Check sheet for the modelled part. Datum: model origin and axes. Units: mm. A direction names the side the tool comes from. Round coordinates to 2 decimals unless told otherwise and drop trailing zeros. Write each loop counter-clockwise with the first axis right and the second up, starting at its lowest first coordinate (ties: lowest second). Pieces come first, ordered by that corner, then holes. Notation, with made-up numbers: (80, 77) -> (106, 77) arc R25 cw to (106, 109) -> close; hole circle Ø1 at (-1.75, 23.25). An arc over 180 degrees is marked (long way). One line per item, written item: value.
from build123d import *

# Parameters (mm, degrees)
SKETCH1_W           = 99.695
SKETCH1_H           = 17.526
BOSS_EXTRUDE1_DEPTH = 2.54
SKETCH2_W           = 104.14
SKETCH2_H           = 20.193
BOSS_EXTRUDE2_DEPTH = 2.54
SKETCH4_W           = 20.32
SKETCH4_H           = 8.89
BOSS_EXTRUDE3_DEPTH = 3.81
SKETCH5_W           = 50.8
SKETCH5_H           = 17.526
CUT_EXTRUDE1_DEPTH  = 54.282554483


with BuildPart() as part:
    # Sketch1 → Boss-Extrude1 (new body)
    with BuildSketch(Plane(origin=(0, 0, 0), x_dir=(1, 0, 0), z_dir=(0, 1, 0))):
        Rectangle(SKETCH1_W, SKETCH1_H)
    extrude(amount=BOSS_EXTRUDE1_DEPTH)

    # Sketch2 → Boss-Extrude2 (add)
    with BuildSketch(Plane(origin=(0, 2.54, 0), x_dir=(1, 0, 0), z_dir=(0, 1, 0))):
        Rectangle(SKETCH2_W, SKETCH2_H)
    extrude(amount=BOSS_EXTRUDE2_DEPTH)

    # Sketch4 → Boss-Extrude3 (add)
    with BuildSketch(Plane(origin=(0, 5.08, 0), x_dir=(1, 0, 0), z_dir=(0, 1, 0))):
        with Locations((28.80358553, 0)):
            Rectangle(SKETCH4_W, SKETCH4_H)
    extrude(amount=BOSS_EXTRUDE3_DEPTH)

    # Sketch5 → Cut-Extrude1 (cut, through all)
    with BuildSketch(Plane(origin=(0, 5.08, 0), x_dir=(1, 0, 0), z_dir=(0, 1, 0))):
        with Locations((-21.59, 0)):
            Rectangle(SKETCH5_W, SKETCH5_H)
    extrude(amount=-CUT_EXTRUDE1_DEPTH, mode=Mode.SUBTRACT)


solid = part.part
Item 1: Sectioned sample at B-B on x = -41.5. Enter the section's corners in (y, z).
Answer:
outline: (2.54, -10.1) -> (5.08, -10.1) -> (5.08, -8.76) -> (2.54, -8.76) -> close; (2.54, 8.76) -> (5.08, 8.76) -> (5.08, 10.1) -> (2.54, 10.1) -> close
Item 2: Mould release check, pull along Z, two halves, no side actions. Record for faces 1 (the flat face through (29, 7, -4.445)), 2 (the flat face through (-22, 4, 8.763)), 3 (the flat face through (18.644, 7, 0)): pulls with the +Z half, pulls with the -Z half, needs draft (parallel to the pull), parting line crosses it, or undercut.
Answer:
face 1: pulls with the -Z half
face 2: undercut
face 3: needs draft
Item 3: Sectioned sample at A-A on z = -1.25. Enter the section's corners in (x, y), and give its area (3 significant figures).
Answer:
outline: (-52.07, 2.54) -> (-49.85, 2.54) -> (-49.85, 0) -> (-46.99, 0) -> (-46.99, 5.08) -> (-52.07, 5.08) -> close; (3.81, 0) -> (49.85, 0) -> (49.85, 2.54) -> (52.07, 2.54) -> (52.07, 5.08) -> (38.96, 5.08) -> (38.96, 8.89) -> (18.64, 8.89) -> (18.64, 5.08) -> (3.81, 5.08) -> close
area: 337 mm^2
Item 4: Thickness scan on line 1 (X direction, y = 4, z = -8.25); line 2 (Z direction, x = 0, y = 3); line 3 (X direction, y = 2.25, z = 6.25). Record the ranges inside material, lowest first.
Answer:
line 1: x = -52.07 to -46.99, 3.81 to 52.07
line 2: z = -10.1 to -8.76, 8.76 to 10.1
line 3: x = -49.85 to -46.99, 3.81 to 49.85
Item 5: Sectioned sample at C-C on z = -5.5. Enter the section's corners in (x, y), and give its area (3 significant figures).
Answer:
outline: (-52.07, 2.54) -> (-49.85, 2.54) -> (-49.85, 0) -> (-46.99, 0) -> (-46.99, 5.08) -> (-52.07, 5.08) -> close; (3.81, 0) -> (49.85, 0) -> (49.85, 2.54) -> (52.07, 2.54) -> (52.07, 5.08) -> (3.81, 5.08) -> close
area: 260 mm^2
Item 6: Sectioned sample at D-D on x = 24.5. Enter the section's corners in (y, z) (1 decimal).
Answer:
outline: (0, -8.8) -> (2.5, -8.8) -> (2.5, -10.1) -> (5.1, -10.1) -> (5.1, -4.4) -> (8.9, -4.4) -> (8.9, 4.4) -> (5.1, 4.4) -> (5.1, 10.1) -> (2.5, 10.1) -> (2.5, 8.8) -> (0, 8.8) -> close
Item 7: Depth check by flat-ended pin: P1, Ø3, axis at x = 27, y = 7.5, coming from the +Z side (3 decimals); P2, Ø1.5, axis at x = -15.5, z = -6.5, coming from the -Y side; P3, Ø2, axis at x = -49, y = 1, coming from the +Z side; P4, Ø3, axis at x = 32, y = 7.5, coming from the -Z side (3 decimals). Enter the tip coordinate at first touch or a pass-through.
Answer:
P1: stops at z = 4.445
P2: passes through
P3: stops at z = 8.76
P4: stops at z = -4.445
Item 8: Tool access check on faces 4 (the flat face through (29, 7, 4.445)), 5 (the flat face through (3.81, 3, 0)), 6 (the flat face through (27, 1, 8.763)). Record the directions out of +Z, -Z, +X, -X, +Y, -Y that give a thin tool (end or side, any length) a straight path to the whole face; none if there is none.
Answer:
face 4: +Z, +X, -X, +Y
face 5: +Y, -Y
face 6: +Z, +X, -X, -Y
